CAD build for the part. Positions are in the model's coordinates, mm. Face numbers are marked on the shaded views. A direction names the side the tool comes from. Coordinates: 2 decimals unless noted, no trailing zeros. Loops run counter-clockwise (first coordinate to the right, second up) from the corner with the lowest first, then second, coordinate; pieces in that order, holes last. Notation, with made-up numbers: (17, -28.75) -> (24, -28.75) arc R5 cw to (24, -20.75) -> close; hole circle Ø9 at (-24, 25). An arc over 180 degrees is marked (long way). Write item = value, one per line. Start each with the question number.
(1) Flat gauge pins, fed straight in: P1, Ø8, axis at x = 4, z = -13.5, coming from the -Y side; P2, Ø2, axis at x = 6.5, z = 22.5, coming from the +Y side; P3, Ø4, axis at x = -4, y = -4, coming from the +Z side. Where does each tip first touch, or does it go through?
(2) Band-saw the part on C-C (x = -0.25). Write the cut outline in (y, z), and give its area (3 significant figures).
(3) Pull direction Y, two halves, no side cores. Call the marked faces 1, 2 and 3: +Y half, -Y half, draft (parallel to the pull), parting line (faces both ways), or undercut.
(4) Band-saw the part on D-D (x = -4). Write the cut outline in (y, z) (3 decimals).
(5) Tool access for the marked faces 4, 5 and 6: list every direction of +Z, -Z, +X, -X, +Y, -Y with a clear straight run to the whole face (end or side of a thin tool).
(6) Drill centre lines: line 1 (Y direction, x = 1.25, z = 0); line 2 (X direction, y = -17, z = -6.5); line 3 (X direction, y = 9, z = -25). Where is each one in solid material? Low to high. Write a range as from..to.
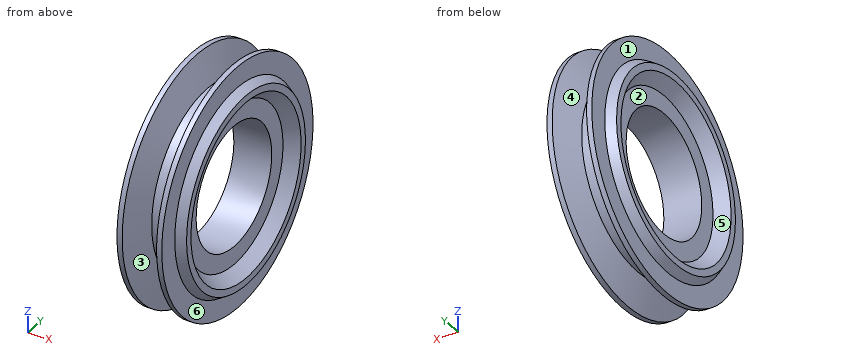
```python
from build123d import *

# Parameters (mm, degrees)
SKETCH_2_R          = 17.5
CUT_EXTRUDE_1_DEPTH = 52.577611422
SKETCH_4_W          = 5.67471706
SKETCH_4_H          = 4.873840026


with BuildPart() as part:
    # Эскиз1 → Повернуть1 (revolve)
    with BuildSketch(Plane.XY, mode=Mode.PRIVATE) as revolve_1_sk:
        Polygon((5.5, 0), (5.5, 22.7), (9, 25.5), (9, 27.5), (6.5, 29), (6.5, 35), (5, 35), (1, 22.7), (-1, 22.7), (-5, 35), (-6.5, 35), (-6.5, 29), (-9, 27.5), (-9, 25.5), (-5.5, 22.7), (-5.5, 0), align=None)
    revolve(revolve_1_sk.sketch.rotate(Axis((-55.549199464, 0, 0), (1, 0, 0)), 90), axis=Axis((-55.549199464, 0, 0), (1, 0, 0)))

    # Эскиз2 → Вырез-Вытянуть1 (cut, through all)
    with BuildSketch(Plane(origin=(5.5, 0, 0), x_dir=(0, 0, -1), z_dir=(1, 0, 0))):
        Circle(SKETCH_2_R)
    extrude(amount=-CUT_EXTRUDE_1_DEPTH, mode=Mode.SUBTRACT)

    # Эскиз4 → Повернуть2 (revolve)
    with BuildSketch(Plane.XY, mode=Mode.PRIVATE) as revolve_2_sk:
        with Locations((0, 23.563079987)):
            Rectangle(SKETCH_4_W, SKETCH_4_H)
    revolve(revolve_2_sk.sketch.rotate(Axis((-55.549199464, 0, 0), (1, 0, 0)), 90), axis=Axis((-55.549199464, 0, 0), (1, 0, 0)))


solid = part.part
```
Findings below:
q1.P1 = -33.65
q1.P2 = 27.62
q1.P3 = 34.93
q2.outline = circle Ø52 at (0, 0); hole circle Ø35 at (0, 0)
q2.area = 1,160 mm²
q3.face_1 = draft
q3.face_2 = undercut
q3.face_3 = parting line
q4.outline = circle Ø63.85 at (0, 0); hole circle Ø35 at (0, 0)
q5.face_4 = none
q5.face_5 = -X
q5.face_6 = +X
q6.line_1 = -26..-17.5, 17.5..26
q6.line_2 = -5.5..5.5
q6.line_3 = -9..-2.26, 2.26..9
